```python
from build123d import *

# Parameters (mm, degrees)
SKETCH2_W           = 43
SKETCH2_H           = 43
BOSS_EXTRUDE1_DEPTH = 2
CUT_EXTRUDE1_REACH  = 62.844
SKETCH3_R           = 1.5
CUT_EXTRUDE2_REACH  = 62.844
SKETCH4_R           = 1.5
SKETCH5_W           = 21
SKETCH5_H           = 15
BOSS_EXTRUDE2_DEPTH = 5
SKETCH6_W           = 15
SKETCH6_H           = 11
BOSS_EXTRUDE3_DEPTH = 2.5
SKETCH7_W           = 21
SKETCH7_H           = 7
CUT_EXTRUDE3_DEPTH  = 2.5


with BuildPart() as part:
    # Sketch2 → Boss-Extrude1 (new body)
    with BuildSketch(Plane.XY):
        with Locations((21.5, 21.5)):
            Rectangle(SKETCH2_W, SKETCH2_H)
    extrude(amount=BOSS_EXTRUDE1_DEPTH)

    # Sketch3 → Cut-Extrude1 (cut, up to next)
    with BuildSketch(Plane.XY.offset(2), mode=Mode.PRIVATE) as cut_extrude1_sk1:
        with Locations((6.5, 36.5)):
            Circle(SKETCH3_R)
    cut_extrude1_tool1 = extrude(cut_extrude1_sk1.sketch, amount=-CUT_EXTRUDE1_REACH, mode=Mode.PRIVATE) & part.part
    add(cut_extrude1_tool1.solids().sort_by_distance((6.5, 36.5, 2))[0], mode=Mode.SUBTRACT)

    # Sketch4 → Cut-Extrude2 (cut, up to next)
    with BuildSketch(Plane.XY.offset(2), mode=Mode.PRIVATE) as cut_extrude2_sk1:
        with Locations((36.5, 6.5)):
            Circle(SKETCH4_R)
    cut_extrude2_tool1 = extrude(cut_extrude2_sk1.sketch, amount=-CUT_EXTRUDE2_REACH, mode=Mode.PRIVATE) & part.part
    add(cut_extrude2_tool1.solids().sort_by_distance((36.5, 6.5, 2))[0], mode=Mode.SUBTRACT)

    # Sketch5 → Boss-Extrude2 (add)
    with BuildSketch(Plane.XY.offset(2)):
        with Locations((25.5, 42.5)):
            Rectangle(SKETCH5_W, SKETCH5_H)
    extrude(amount=BOSS_EXTRUDE2_DEPTH)

    # Sketch6 → Boss-Extrude3 (add)
    with BuildSketch(Plane.XY.offset(2)):
        with Locations((0.5, 17.5)):
            Rectangle(SKETCH6_W, SKETCH6_H)
    extrude(amount=BOSS_EXTRUDE3_DEPTH)

    # Sketch7 → Cut-Extrude3 (cut)
    with BuildSketch(Plane(origin=(0, 0, 2), x_dir=(-1, 0, 0), z_dir=(0, 0, -1))):
        with Locations((-25.5, 46.5)):
            Rectangle(SKETCH7_W, SKETCH7_H)
    extrude(amount=-CUT_EXTRUDE3_DEPTH, mode=Mode.SUBTRACT)


solid = part.part
```
Can you work these out from the model? Positions are in its coordinate system, mm. A direction names the side the tool comes from. Give positions to 0.01 mm unless a question says otherwise; leave off trailing zeros. Loops run counter-clockwise (first coordinate to the right, second up) from the corner with the lowest first, then second, coordinate; pieces in that order, holes last. Notation, with made-up numbers: M 50,6 L 54,6 A21 cw 54,30 Z; hole C 68,31.5 d10. An arc over 180 degrees is marked long. Use one line per item in the form item = value. Start each with the question number.
(1) I want a section at B-B, the plane y = 36.5. Write out the boundary of the cut face in (x, z), and give its area (3 significant figures).
(2) I'm going to push flat-ended pins straight in: P1, Ø10, axis at x = 29, y = 12.5, coming from the +Z side; P2, Ø4, axis at x = 8, z = 1.5, coming from the +Y side; P3, Ø1, axis at y = 35, z = 5.5, coming from the -X side; P4, Ø4, axis at x = 6.5, y = 36.5, coming from the -Z side. Where does each tip first touch, or does it pass through?
(3) Please list where these lines run through material, in increasing order: line 1 (Y direction, x = 36.5, z = 0.9); line 2 (Y direction, x = 6.5, z = 1.25); line 3 (X direction, y = 15.5, z = 1).
(4) On a 3-axis mill with a long thin cutter (end or side, diameter ignored), from which of +Z, -Z, +X, -X, +Y, -Y can I reach the whole of each face in a straight line? I mean faces 1 (the flat face through (-4, 18, 2)), 2 (the flat face through (15, 41, 5)), 3 (the flat face through (26, 47, 4.5)), 4 (the flat face through (0, 12, 3)). Say none if no direction works.
(5) I want a section at A-A, the plane x = 6.5. Write out the boundary of the cut face in (y, z).
(6) I want a section at C-C, the plane x = 22.5. Write out the boundary of the cut face in (y, z), and give its area (4 significant figures).
(7) I want a section at D-D, the plane y = 19. Write out the boundary of the cut face in (x, z), and give its area (4 significant figures).
Worked out:
q1.outline = M 0,0 L 5,0 L 5,2 L 0,2 Z; M 8,0 L 43,0 L 43,2 L 36,2 L 36,7 L 15,7 L 15,2 L 8,2 Z
q1.area = 185 mm²
q2.P1 = 2
q2.P2 = 43
q2.P3 = 15
q2.P4 = 0
q3.line_1 = 0 to 5, 8 to 43
q3.line_2 = 0 to 35, 38 to 43
q3.line_3 = 0 to 43
q4.face_1 = -Z, -X, +Y, -Y
q4.face_2 = +Z, -X, +Y, -Y
q4.face_3 = -Z, +X, -X, +Y
q4.face_4 = +Z, +X, -X, -Y
q5.outline = M 0,0 L 35,0 L 35,2 L 23,2 L 23,4.5 L 12,4.5 L 12,2 L 0,2 Z; M 38,0 L 43,0 L 43,2 L 38,2 Z
q6.outline = M 0,0 L 43,0 L 43,4.5 L 50,4.5 L 50,7 L 35,7 L 35,2 L 0,2 Z
q6.area = 143.5 mm²
q7.outline = M -7,2 L 0,2 L 0,0 L 43,0 L 43,2 L 8,2 L 8,4.5 L -7,4.5 Z
q7.area = 123.5 mm²
